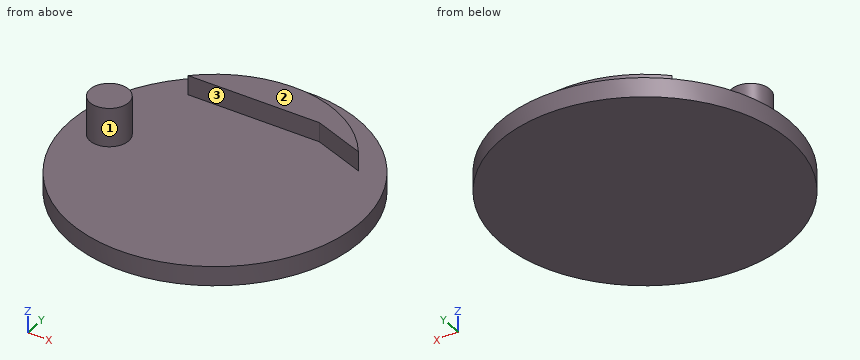
```python
from build123d import *

# Parameters (mm, degrees)
SKETCH1_R           = 37.5
BOSS_EXTRUDE1_DEPTH = 5
BOSS_EXTRUDE2_DEPTH = 5
SKETCH4_R           = 5
BOSS_EXTRUDE3_DEPTH = 10


with BuildPart() as part:
    # Sketch1 → Boss-Extrude1 (new body)
    with BuildSketch(Plane.XY):
        Circle(SKETCH1_R)
    extrude(amount=BOSS_EXTRUDE1_DEPTH)

    # Sketch3 → Boss-Extrude2 (add)
    with BuildSketch(Plane.XY.offset(5)):
        with BuildLine():
            Line((25.890393972, 17.5), (12.5, 22.5))
            Line((12.5, 22.5), (-21.686689466, 22.5))
            ThreePointArc((-21.686689466, 22.5), (3.266157206, 31.078846779), (25.890393972, 17.5))
        make_face()
    extrude(amount=BOSS_EXTRUDE2_DEPTH)

    # Sketch4 → Boss-Extrude3 (add)
    with BuildSketch(Plane.XY.offset(5)):
        with Locations((-27.5, 0)):
            Circle(SKETCH4_R)
    extrude(amount=BOSS_EXTRUDE3_DEPTH)


solid = part.part
```
Verification items for the finished model (mm, model axes). Face numbers are marked on the shaded views. A direction names the side the tool comes from. Coordinates: 2 decimals unless noted, no trailing zeros. Loops run counter-clockwise (first coordinate to the right, second up) from the corner with the lowest first, then second, coordinate; pieces in that order, holes last. Notation, with made-up numbers: (51, -15) - (78, -15) arc R36 cw to (78, 22) - close; hole circle Ø6 at (52, 61.5). An arc over 180 degrees is marked (long way). Return JSON: item names as keys, results as strings.
1. Section check B-B, the plane y = 0. Record the boundary of the cut face in (x, z).
Established:
{"outline": "(-37.5, 0) - (37.5, 0) - (37.5, 5) - (-22.5, 5) - (-22.5, 15) - (-32.5, 15) - (-32.5, 5) - (-37.5, 5) - close"}
2. Section check A-A, the plane x = 0. Record the boundary of the cut face in (y, z), then the cut area to 3 significant figures.
Established:
{"outline": "(-37.5, 0) - (37.5, 0) - (37.5, 5) - (31.25, 5) - (31.25, 10) - (22.5, 10) - (22.5, 5) - (-37.5, 5) - close", "area": "419 mm2"}
3. Go/stop test with flat-tipped pins: pin 1 (4 mm diameter, centred on x = -2, z = 7.5, fed in from -Y); pin 2 (1.5 mm diameter, centred on x = 15, z = 9, fed in from +Y); pin 3 (15 mm diameter, centred on x = 9, y = 27, fed in from +Z). Record where each tip stops, or that it passes through.
Established:
{"pin 1": "stops at y = 22.5", "pin 2": "stops at y = 27.81", "pin 3": "stops at z = 10"}
4. Section check D-D, the plane y = -8.5. Record the boundary of the cut face in (x, z).
Established:
{"outline": "(-36.52, 0) - (36.52, 0) - (36.52, 5) - (-36.52, 5) - close"}
5. Section check C-C, the plane z = 1. Record the boundary of the cut face in (x, y), then the cut area to 3 significant figures.
Established:
{"outline": "circle Ø75 at (0, 0)", "area": "4,420 mm2"}
6. Thickness scan on L1, parallel to Z at x = -29, y = -5; L2, parallel to Z at x = -11, y = 25; L3, parallel to Y at x = -24, z = 7. Record the ranges inside material, lowest first.
Established:
{"L1": "z = 0 to 5", "L2": "z = 0 to 10", "L3": "y = -3.57 to 3.57"}
7. Tool access check on the marked faces 1, 2 and 3. Record the directions out of +Z, -Z, +X, -X, +Y, -Y that give a thin tool (end or side, any length) a straight path to the whole face; none if there is none.
Established:
{"face 1": "+Z", "face 2": "+Z, +X, -X, +Y, -Y", "face 3": "+Z, -X, -Y"}
